Work out the finished part from the listing and answer in its coordinate system (mm). A direction names the side the tool comes from. Coordinates: 2 decimals unless noted, no trailing zeros. Order: outer loops, then holes, each group sorted by start corner. A loop starts at its lowest first (then second) coordinate and runs counter-clockwise, first axis right, second up.
1. Determine the mould class of faces 4 (the flat face through (-3, 190.5, 132)), 5 (the flat face through (-222.25, -3, 125)), 6 (the flat face through (-18, -195, 254)) for opening direction X: +X half, -X half, draft (parallel to the pull), parting line (faces both ways), or undercut.
2. Find the intervals of material crossed by probe 1 along X at (y, z) = (-16.5, 67.5); probe 2 along Y at (x, z) = (-61, 187); probe 3 along Z at (x, y) = (-174.5, -128.5), in increasing order.
3. The part is cut by section A-A, the plane z = 190. Give the vertices of the cut face in (x, y), then the cut area to 3 significant figures.
4. The part is cut by section C-C, the plane x = -70. Give the vertices of the cut face in (y, z), then the cut area to 3 significant figures.
5. Flat-ended cylindrical pins translate along their axes: pin 1 Ø4 at (x, y) = (-135.5, -58) entering from -Z; pin 2 Ø1 at (x, y) = (115.5, -26.5) entering from +Z. Find the tip coordinate at first contact, or state that the pin passes through.
6. The part is cut by section B-B, the plane y = 111. Give the vertices of the cut face in (x, z).
7. A tool of negligible diameter and unlimited length cuts with its end or side. For faces 1 (the flat face through (-3, -3, 12.7)), 2 (the flat face through (-3, -3, 6.35)), 3 (the flat face through (-3, -203.2, 125)), from which of +Z, -Z, +X, -X, +Y, -Y can it reach the whole face along a straight path? Write none if from no direction.
```python
from build123d import *

# Parameters (mm, degrees)
F0_W     = 444.5
F0_H     = 406.4
F0_W_2   = 419.1
F0_H_2   = 381
F1_DEPTH = 254
F2_W     = 419.1
F2_H     = 381
F3_DEPTH = 12.7
F4_W     = 419.1
F4_H     = 381
F5_DEPTH = 6.35


with BuildPart() as f1:
    # F0 (on Top) → F1 (new body)
    with BuildSketch(Plane.XY):
        Rectangle(F0_W, F0_H)
        Rectangle(F0_W_2, F0_H_2, mode=Mode.SUBTRACT)
    extrude(amount=F1_DEPTH)

    # F2 (on face) → F3 (join)
    with BuildSketch(Plane(origin=(0, 0, 0), x_dir=(1, 0, 0), z_dir=(0, 0, -1))):
        Rectangle(F2_W, F2_H)
    extrude(amount=-F3_DEPTH)

    # F4 (on face) → F5 (cut)
    with BuildSketch(Plane(origin=(0, 0, 0), x_dir=(1, 0, 0), z_dir=(0, 0, -1))):
        Rectangle(F4_W, F4_H)
    extrude(amount=-F5_DEPTH, mode=Mode.SUBTRACT)


solid = f1.part
```
Geometry says:
1. face 4: undercut
1. face 5: -X half
1. face 6: draft
2. probe 1: x = -222.25 to -209.55, 209.55 to 222.25
2. probe 2: y = -203.2 to -190.5, 190.5 to 203.2
2. probe 3: z = 6.35 to 12.7
3. outline: (-222.25, -203.2) - (222.25, -203.2) - (222.25, 203.2) - (-222.25, 203.2) - close; hole (-209.55, -190.5) - (209.55, -190.5) - (209.55, 190.5) - (-209.55, 190.5) - close
3. area: 21,000 mm2
4. outline: (-203.2, 0) - (-190.5, 0) - (-190.5, 6.35) - (190.5, 6.35) - (190.5, 0) - (203.2, 0) - (203.2, 254) - (190.5, 254) - (190.5, 12.7) - (-190.5, 12.7) - (-190.5, 254) - (-203.2, 254) - close
4. area: 8,870 mm2
5. pin 1: stops at z = 6.35
5. pin 2: stops at z = 12.7
6. outline: (-222.25, 0) - (-209.55, 0) - (-209.55, 6.35) - (209.55, 6.35) - (209.55, 0) - (222.25, 0) - (222.25, 254) - (209.55, 254) - (209.55, 12.7) - (-209.55, 12.7) - (-209.55, 254) - (-222.25, 254) - close
7. face 1: +Z
7. face 2: -Z
7. face 3: +Z, -Z, +X, -X, -Y
